Could you check a few things on this model? Use its own coordinates, in mm. Face numbers are marked on the shaded views. A direction names the side the tool comes from. Coordinates: 2 decimals unless noted, no trailing zeros. Loops run counter-clockwise (first coordinate to the right, second up) from the corner with the lowest first, then second, coordinate; pieces in that order, holes last. Notation, with made-up numbers: (-15.5, 44.5) - (35.5, 44.5) arc R12 cw to (35.5, 62.5) - close; hole circle Ø10 at (-19, -4). An arc over 180 degrees is marked (long way). One line per item, written item: value. Start each with the question number.
(1) If we section it at D-D on z = -6.6: Write out the boundary of the cut face in (x, y).
(2) On a 3-axis mill with a long thin cutter (end or side, diameter ignored), from which of +Z, -Z, +X, -X, +Y, -Y can I reach the whole of each face in a straight line? I mean the marked faces 1 and 2. Say none if no direction works.
(3) If we section it at C-C on z = 20.5: Write out the boundary of the cut face in (x, y).
(4) If we section it at A-A on y = 4: Write out the boundary of the cut face in (x, z), then the cut area to 3 significant figures.
(5) I'm going to push flat-ended pins straight in: P1, Ø2, axis at y = 5.5, z = 16, coming from the +X side; P2, Ø2.5, axis at y = 5.5, z = 18, coming from the -X side; P3, Ø1.6, axis at x = -6.85, z = -6.6, coming from the -Y side; P4, Ø1, axis at x = 5, y = 1.5, coming from the -Z side. Where does each tip first touch, or does it pass through?
(6) If I drill on line 1 along X through (y, z) = (0.75, 12.3); line 2 along X through (y, z) = (0.25, -6.6); line 3 along Z through (x, y) = (3.9, 0.2), over which ranges is the centre line in solid material (lowest first)? Write a range as from..to.
(7) If we mould it in two halves opening along X, with no side actions, what happens to the marked faces 3, 4 and 5? For each: pulls with the +X half, pulls with the -X half, needs draft (parallel to the pull), parting line crosses it, or undercut.
(8) If we section it at B-B on z = -17.05: Write out the boundary of the cut face in (x, y).
```python
from build123d import *

# Parameters (mm, degrees)
SKETCH1_W               = 22
SKETCH1_H               = 52
BOSS_EXTRUDE1_DEPTH     = 7
SKETCH2_W               = 20.1
SKETCH2_H               = 50.1
CUT_EXTRUDE1_DEPTH      = 6
SKETCH7_R               = 0.8
CUT_EXTRUDE6_DEPTH      = 7
CUT_EXTRUDE6_DEPTH_BACK = 2
CUT_EXTRUDE7_REACH      = 3
SKETCH8_R               = 1
CUT_EXTRUDE9_REACH      = 3
SKETCH9_R               = 1
CUT_EXTRUDE10_REACH     = 3
SKETCH10_R              = 1
CUT_EXTRUDE11_REACH     = 3
SKETCH11_R              = 1
CUT_EXTRUDE12_REACH     = 3
SKETCH12_R              = 1
CUT_EXTRUDE13_REACH     = 3
SKETCH13_R              = 1
CUT_EXTRUDE14_REACH     = 3
SKETCH14_R              = 1
CUT_EXTRUDE15_REACH     = 3
SKETCH15_R              = 1
CUT_EXTRUDE16_REACH     = 3
SKETCH16_R              = 1
SKETCH18_W              = 2.91
SKETCH18_H              = 52
BOSS_EXTRUDE2_DEPTH     = 2
SKETCH18_3_W            = 2.9
SKETCH18_3_H            = 52
BOSS_EXTRUDE3_DEPTH     = 2
SKETCH19_W              = 10
SKETCH19_H              = 5
CUT_EXTRUDE17_DEPTH     = 25.9


with BuildPart() as part:
    # Sketch1 → Boss-Extrude1 (new body)
    with BuildSketch(Plane(origin=(0, 0, 0), x_dir=(1, 0, 0), z_dir=(0, 1, 0))):
        Rectangle(SKETCH1_W, SKETCH1_H)
    extrude(amount=BOSS_EXTRUDE1_DEPTH)

    # Sketch2 → Cut-Extrude1 (cut)
    with BuildSketch(Plane(origin=(0, 7, 0), x_dir=(1, 0, 0), z_dir=(0, 1, 0))):
        Rectangle(SKETCH2_W, SKETCH2_H)
    extrude(amount=-CUT_EXTRUDE1_DEPTH, mode=Mode.SUBTRACT)

    # Sketch7 → Cut-Extrude6 (cut, two sides)
    with BuildSketch(Plane(origin=(0, 1, 0), x_dir=(1, 0, 0), z_dir=(0, 1, 0))) as cut_extrude6_sk:
        with Locations((-8.15, -23)):
            Circle(SKETCH7_R)
    extrude(amount=CUT_EXTRUDE6_DEPTH, mode=Mode.SUBTRACT)
    extrude(cut_extrude6_sk.sketch, amount=-CUT_EXTRUDE6_DEPTH_BACK, mode=Mode.SUBTRACT)

    # Sketch8 → Cut-Extrude7 (cut, up to next)
    with BuildSketch(Plane(origin=(0, 1, 0), x_dir=(1, 0, 0), z_dir=(0, 1, 0)), mode=Mode.PRIVATE) as cut_extrude7_sk1:
        with Locations((-5.75, -12.3)):
            Circle(SKETCH8_R)
    cut_extrude7_tool1 = extrude(cut_extrude7_sk1.sketch, amount=-CUT_EXTRUDE7_REACH, mode=Mode.PRIVATE) & part.part
    add(cut_extrude7_tool1.solids().sort_by_distance((-5.75, 1, 12.3))[0], mode=Mode.SUBTRACT)
    # Sketch8 → Cut-Extrude7 (cut, up to next)
    with BuildSketch(Plane(origin=(0, 1, 0), x_dir=(1, 0, 0), z_dir=(0, 1, 0)), mode=Mode.PRIVATE) as cut_extrude7_sk2:
        with Locations((5, -12.3)):
            Circle(SKETCH8_R)
    cut_extrude7_tool2 = extrude(cut_extrude7_sk2.sketch, amount=-CUT_EXTRUDE7_REACH, mode=Mode.PRIVATE) & part.part
    add(cut_extrude7_tool2.solids().sort_by_distance((5, 1, 12.3))[0], mode=Mode.SUBTRACT)

    # Sketch9 → Cut-Extrude9 (cut, up to next)
    with BuildSketch(Plane(origin=(0, 1, 0), x_dir=(1, 0, 0), z_dir=(0, 1, 0)), mode=Mode.PRIVATE) as cut_extrude9_sk1:
        with Locations((-5.75, -9.5)):
            Circle(SKETCH9_R)
    cut_extrude9_tool1 = extrude(cut_extrude9_sk1.sketch, amount=-CUT_EXTRUDE9_REACH, mode=Mode.PRIVATE) & part.part
    add(cut_extrude9_tool1.solids().sort_by_distance((-5.75, 1, 9.5))[0], mode=Mode.SUBTRACT)
    # Sketch9 → Cut-Extrude9 (cut, up to next)
    with BuildSketch(Plane(origin=(0, 1, 0), x_dir=(1, 0, 0), z_dir=(0, 1, 0)), mode=Mode.PRIVATE) as cut_extrude9_sk2:
        with Locations((5, -9.5)):
            Circle(SKETCH9_R)
    cut_extrude9_tool2 = extrude(cut_extrude9_sk2.sketch, amount=-CUT_EXTRUDE9_REACH, mode=Mode.PRIVATE) & part.part
    add(cut_extrude9_tool2.solids().sort_by_distance((5, 1, 9.5))[0], mode=Mode.SUBTRACT)

    # Sketch10 → Cut-Extrude10 (cut, up to next)
    with BuildSketch(Plane(origin=(0, 1, 0), x_dir=(1, 0, 0), z_dir=(0, 1, 0)), mode=Mode.PRIVATE) as cut_extrude10_sk1:
        with Locations((-5.75, -6.8)):
            Circle(SKETCH10_R)
    cut_extrude10_tool1 = extrude(cut_extrude10_sk1.sketch, amount=-CUT_EXTRUDE10_REACH, mode=Mode.PRIVATE) & part.part
    add(cut_extrude10_tool1.solids().sort_by_distance((-5.75, 1, 6.8))[0], mode=Mode.SUBTRACT)
    # Sketch10 → Cut-Extrude10 (cut, up to next)
    with BuildSketch(Plane(origin=(0, 1, 0), x_dir=(1, 0, 0), z_dir=(0, 1, 0)), mode=Mode.PRIVATE) as cut_extrude10_sk2:
        with Locations((5, -6.837159935)):
            Circle(SKETCH10_R)
    cut_extrude10_tool2 = extrude(cut_extrude10_sk2.sketch, amount=-CUT_EXTRUDE10_REACH, mode=Mode.PRIVATE) & part.part
    add(cut_extrude10_tool2.solids().sort_by_distance((5, 1, 6.83716))[0], mode=Mode.SUBTRACT)

    # Sketch11 → Cut-Extrude11 (cut, up to next)
    with BuildSketch(Plane(origin=(0, 1, 0), x_dir=(1, 0, 0), z_dir=(0, 1, 0)), mode=Mode.PRIVATE) as cut_extrude11_sk1:
        with Locations((-0.3, -12.3)):
            Circle(SKETCH11_R)
    cut_extrude11_tool1 = extrude(cut_extrude11_sk1.sketch, amount=-CUT_EXTRUDE11_REACH, mode=Mode.PRIVATE) & part.part
    add(cut_extrude11_tool1.solids().sort_by_distance((-0.3, 1, 12.3))[0], mode=Mode.SUBTRACT)

    # Sketch12 → Cut-Extrude12 (cut, up to next)
    with BuildSketch(Plane(origin=(0, 1, 0), x_dir=(1, 0, 0), z_dir=(0, 1, 0)), mode=Mode.PRIVATE) as cut_extrude12_sk1:
        with Locations((3.95, 12.05)):
            Circle(SKETCH12_R)
    cut_extrude12_tool1 = extrude(cut_extrude12_sk1.sketch, amount=-CUT_EXTRUDE12_REACH, mode=Mode.PRIVATE) & part.part
    add(cut_extrude12_tool1.solids().sort_by_distance((3.95, 1, -12.05))[0], mode=Mode.SUBTRACT)
    # Sketch12 → Cut-Extrude12 (cut, up to next)
    with BuildSketch(Plane(origin=(0, 1, 0), x_dir=(1, 0, 0), z_dir=(0, 1, 0)), mode=Mode.PRIVATE) as cut_extrude12_sk2:
        with Locations((-6.8, 12.05)):
            Circle(SKETCH12_R)
    cut_extrude12_tool2 = extrude(cut_extrude12_sk2.sketch, amount=-CUT_EXTRUDE12_REACH, mode=Mode.PRIVATE) & part.part
    add(cut_extrude12_tool2.solids().sort_by_distance((-6.8, 1, -12.05))[0], mode=Mode.SUBTRACT)

    # Sketch13 → Cut-Extrude13 (cut, up to next)
    with BuildSketch(Plane(origin=(0, 1, 0), x_dir=(1, 0, 0), z_dir=(0, 1, 0)), mode=Mode.PRIVATE) as cut_extrude13_sk1:
        with Locations((3.95, 9.3)):
            Circle(SKETCH13_R)
    cut_extrude13_tool1 = extrude(cut_extrude13_sk1.sketch, amount=-CUT_EXTRUDE13_REACH, mode=Mode.PRIVATE) & part.part
    add(cut_extrude13_tool1.solids().sort_by_distance((3.95, 1, -9.3))[0], mode=Mode.SUBTRACT)
    # Sketch13 → Cut-Extrude13 (cut, up to next)
    with BuildSketch(Plane(origin=(0, 1, 0), x_dir=(1, 0, 0), z_dir=(0, 1, 0)), mode=Mode.PRIVATE) as cut_extrude13_sk2:
        with Locations((-6.8, 9.3)):
            Circle(SKETCH13_R)
    cut_extrude13_tool2 = extrude(cut_extrude13_sk2.sketch, amount=-CUT_EXTRUDE13_REACH, mode=Mode.PRIVATE) & part.part
    add(cut_extrude13_tool2.solids().sort_by_distance((-6.8, 1, -9.3))[0], mode=Mode.SUBTRACT)

    # Sketch14 → Cut-Extrude14 (cut, up to next)
    with BuildSketch(Plane(origin=(0, 1, 0), x_dir=(1, 0, 0), z_dir=(0, 1, 0)), mode=Mode.PRIVATE) as cut_extrude14_sk1:
        with Locations((3.9, 6.6)):
            Circle(SKETCH14_R)
    cut_extrude14_tool1 = extrude(cut_extrude14_sk1.sketch, amount=-CUT_EXTRUDE14_REACH, mode=Mode.PRIVATE) & part.part
    add(cut_extrude14_tool1.solids().sort_by_distance((3.9, 1, -6.6))[0], mode=Mode.SUBTRACT)
    # Sketch14 → Cut-Extrude14 (cut, up to next)
    with BuildSketch(Plane(origin=(0, 1, 0), x_dir=(1, 0, 0), z_dir=(0, 1, 0)), mode=Mode.PRIVATE) as cut_extrude14_sk2:
        with Locations((-6.85, 6.6)):
            Circle(SKETCH14_R)
    cut_extrude14_tool2 = extrude(cut_extrude14_sk2.sketch, amount=-CUT_EXTRUDE14_REACH, mode=Mode.PRIVATE) & part.part
    add(cut_extrude14_tool2.solids().sort_by_distance((-6.85, 1, -6.6))[0], mode=Mode.SUBTRACT)

    # Sketch15 → Cut-Extrude15 (cut, up to next)
    with BuildSketch(Plane(origin=(0, 1, 0), x_dir=(1, 0, 0), z_dir=(0, 1, 0)), mode=Mode.PRIVATE) as cut_extrude15_sk1:
        with Locations((-1.6, 11.05)):
            Circle(SKETCH15_R)
    cut_extrude15_tool1 = extrude(cut_extrude15_sk1.sketch, amount=-CUT_EXTRUDE15_REACH, mode=Mode.PRIVATE) & part.part
    add(cut_extrude15_tool1.solids().sort_by_distance((-1.6, 1, -11.05))[0], mode=Mode.SUBTRACT)

    # Sketch16 → Cut-Extrude16 (cut, up to next)
    with BuildSketch(Plane(origin=(0, 1, 0), x_dir=(1, 0, 0), z_dir=(0, 1, 0)), mode=Mode.PRIVATE) as cut_extrude16_sk1:
        with Locations((-8.25, 17.05)):
            Circle(SKETCH16_R)
    cut_extrude16_tool1 = extrude(cut_extrude16_sk1.sketch, amount=-CUT_EXTRUDE16_REACH, mode=Mode.PRIVATE) & part.part
    add(cut_extrude16_tool1.solids().sort_by_distance((-8.25, 1, -17.05))[0], mode=Mode.SUBTRACT)

    # Sketch18 → Boss-Extrude2 (add)
    with BuildSketch(Plane.XZ):
        with Locations((-12.455, 0)):
            Rectangle(SKETCH18_W, SKETCH18_H)
    extrude(amount=-BOSS_EXTRUDE2_DEPTH)

    # Sketch18<3> → Boss-Extrude3 (add)
    with BuildSketch(Plane.XZ):
        with Locations((12.45, -0.012983648)):
            Rectangle(SKETCH18_3_W, SKETCH18_3_H)
    extrude(amount=-BOSS_EXTRUDE3_DEPTH)

    # Sketch19 → Cut-Extrude17 (cut, through all)
    with BuildSketch(Plane.ZY.offset(11)):
        with Locations((0, 4.5)):
            Rectangle(SKETCH19_W, SKETCH19_H)
    extrude(amount=-CUT_EXTRUDE17_DEPTH, mode=Mode.SUBTRACT)


solid = part.part
```
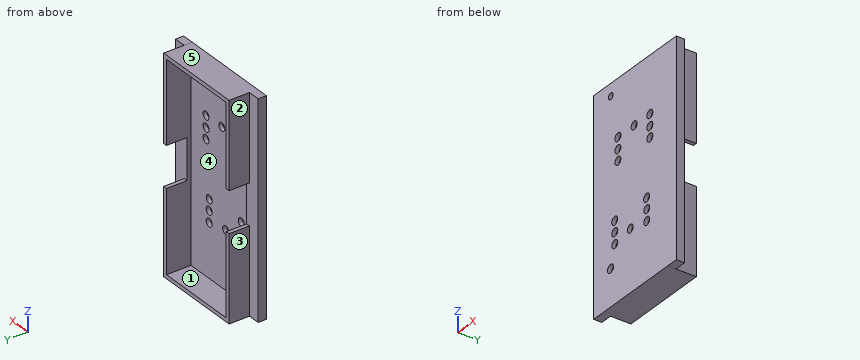
Values:
1. outline: (-13.91, 0) - (-7.85, 0) - (-7.85, 1) - (-10.05, 1) - (-10.05, 7) - (-11, 7) - (-11, 2) - (-13.91, 2) - close; (-5.85, 0) - (2.9, 0) - (2.9, 1) - (-5.85, 1) - close; (4.9, 0) - (13.9, 0) - (13.9, 2) - (11, 2) - (11, 7) - (10.05, 7) - (10.05, 1) - (4.9, 1) - close
2. face 1: +Y
2. face 2: +Z, -Z, -X, +Y
3. outline: (-13.91, 0) - (13.9, 0) - (13.9, 2) - (11, 2) - (11, 7) - (10.05, 7) - (10.05, 1) - (-10.05, 1) - (-10.05, 7) - (-11, 7) - (-11, 2) - (-13.91, 2) - close
4. outline: (-11, -26) - (11, -26) - (11, -5) - (10.05, -5) - (10.05, -25.05) - (-10.05, -25.05) - (-10.05, -5) - (-11, -5) - close; (-11, 5) - (-10.05, 5) - (-10.05, 25.05) - (10.05, 25.05) - (10.05, 5) - (11, 5) - (11, 26) - (-11, 26) - close
4. area: 118 mm2
5. P1: stops at x = 11
5. P2: stops at x = -11
5. P3: passes through
5. P4: stops at z = -26
6. line 1: x = -13.91..-6.75, -4.75..-1.3, 0.7..4, 6..13.9
6. line 2: x = -13.91..-7.85, -5.85..2.9, 4.9..13.9
6. line 3: z = -26..-13.05, -11.05..-10.3, -8.3..-7.6, -5.6..26
7. face 3: pulls with the -X half
7. face 4: undercut
7. face 5: needs draft
8. outline: (-13.91, 0) - (-9.25, 0) - (-9.25, 1) - (-10.05, 1) - (-10.05, 7) - (-11, 7) - (-11, 2) - (-13.91, 2) - close; (-7.25, 0) - (13.9, 0) - (13.9, 2) - (11, 2) - (11, 7) - (10.05, 7) - (10.05, 1) - (-7.25, 1) - close
